```python
from build123d import *

# Parameters (mm, degrees)
ESTRUSIONE_ESTRUSIONE1_DEPTH = 50
SMUSSO1_SIZE                 = 2


with BuildPart() as part:
    # Schizzo1 → Estrusione-Estrusione1 (new body)
    with BuildSketch(Plane.XY):
        Polygon((5, 0), (-5, 0), (-5, -17), (-11, -17), (-11, 8), (11, 8), (11, -17), (5, -17), align=None)
    extrude(amount=ESTRUSIONE_ESTRUSIONE1_DEPTH)

    # Smusso1
    smusso1_edges = [part.edges().sort_by_distance(p)[0] for p in [
        (11, -4.5, 0),
        (11, -4.5, 50),
        (-11, -17, 25),
        (11, -17, 25),
        (-11, -4.5, 50),
        (-11, -4.5, 0),
    ]]
    chamfer(smusso1_edges, length=SMUSSO1_SIZE)


solid = part.part
```
Here's how the part is built. I have some questions about the finished solid (model axes, mm). A direction names the side the tool comes from. Round coordinates to 2 decimals unless told otherwise and drop trailing zeros. Write each loop counter-clockwise with the first axis right and the second up, starting at its lowest first coordinate (ties: lowest second). Pieces come first, ordered by that corner, then holes.
Q1. If we mould it in two halves opening along X, with no side actions, what happens to faces 3 (the flat face through (0, 8, 25)), 4 (the flat face through (11, -3, 25)), 5 (the flat face through (5, -9, 25))? For each: +X half, -X half, draft (parallel to the pull), parting line (faces both ways), or undercut.
Q2. If we section it at B-B on z = 41: Write out the boundary of the cut face in (x, y).
Q3. Which directions (+Z, -Z, +X, -X, +Y, -Y) give clear straight access to the entire face, cutting with the end or side of a thin tool? Please do faces 1 (the flat face through (0, 0, 25)), 2 (the flat face through (7, -17, 25)).
Q4. If we section it at C-C on x = 1.25: Write out the boundary of the cut face in (y, z), plus the area to 3 significant figures.
Q5. Will these pins go through, and if not, where does the flat tip stop? P1, Ø4, axis at x = 1.5, z = 15.5, coming from the -Y side; P2, Ø5, axis at x = 3.5, y = -7, coming from the -Z side.
Q6. Please list where these lines run through material, in increasing order: probe 1 along X at (y, z) = (-7.5, 27); probe 2 along Y at (x, z) = (2.25, 37); probe 3 along Y at (x, z) = (10.25, 18).
Q7. If we section it at A-A on y = -9.25: Write out the boundary of the cut face in (x, z).
Answer below:
1. face 3: draft
1. face 4: +X half
1. face 5: undercut
2. outline: (-11, -15) - (-9, -17) - (-5, -17) - (-5, 0) - (5, 0) - (5, -17) - (9, -17) - (11, -15) - (11, 8) - (-11, 8) - close
3. face 1: +Z, -Z, -Y
3. face 2: +Z, -Z, +X, -X, -Y
4. outline: (0, 0) - (8, 0) - (8, 50) - (0, 50) - close
4. area: 400 mm2
5. P1: stops at y = 0
5. P2: stops at z = 0
6. probe 1: x = -11 to -5, 5 to 11
6. probe 2: y = 0 to 8
6. probe 3: y = -15.75 to 8
7. outline: (-11, 2) - (-9, 0) - (-5, 0) - (-5, 50) - (-9, 50) - (-11, 48) - close; (5, 0) - (9, 0) - (11, 2) - (11, 48) - (9, 50) - (5, 50) - close
